Model file for the job. Use its own axes, mm. Face numbers are marked on the shaded views. A direction names the side the tool comes from. Round coordinates to 2 decimals unless told otherwise and drop trailing zeros. Loops run counter-clockwise (first coordinate to the right, second up) from the corner with the lowest first, then second, coordinate; pieces in that order, holes last. Notation, with made-up numbers: (-23, 79) - (33, 79) arc R16 ccw to (33, 98) - close; hole circle Ø4 at (23.5, 1.25). An arc over 180 degrees is marked (long way). Answer as a JSON object with one key per item and string values.
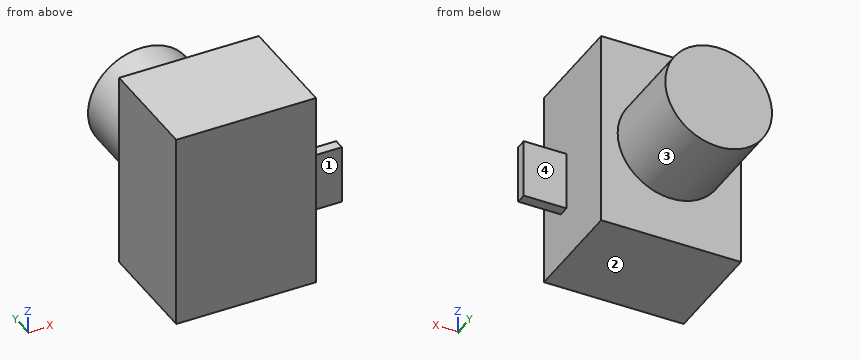
Autodesk Inventor part; units mm, degrees
ref_plane "YZ Plane" through (0, 0, 0) normal (1, 0, 0) x (0, 1, 0)
ref_plane "XZ Plane" through (0, 0, 0) normal (0, 1, 0) x (-1, 0, 0)
ref_plane "XY Plane" through (0, 0, 0) normal (0, 0, 1) x (1, 0, 0)
sketch "Sketch1" plane through (0, 0, 0) normal (0, 1, 0) x (-1, 0, 0)
  line L0 (-6.55, 9.3) -> (6.55, 9.3)
  line L1 (6.55, 9.3) -> (6.55, -9.3)
  line L2 (6.55, -9.3) -> (-6.55, -9.3)
  line L3 (-6.55, -9.3) -> (-6.55, 9.3)
  line L4 (0, 0) -> (1, 0)
  line L5 (0, 0) -> (0, -1)
  dimension "d0" = 18.6
  dimension "d1" = 13.1
  dimension "d2" = 1
  dimension "d3" = 1
extrude "Extrusion1" add sketch "Sketch1" along normal blind 10.2
sketch "Sketch2" plane through (0, 10.2, 0) normal (0, 1, 0) x (1, 0, 0)
  circle A0 centre (0, 0) radius 5
  dimension "d6" = 10
extrude "Extrusion2" add sketch "Sketch2" along normal blind 8.5
sketch "Sketch3" plane through (6.55, 0, 9.3) normal (1, 0, 0) x (0, 0, -1)
  point P0 (9.3, 0)
sketch "Sketch4" plane through (6.55, 0, 9.3) normal (1, 0, 0) x (0, 0, -1)
  circle A0 centre (7.5, 3.5) radius 2.5
  line L0 (0, 0) -> (0, 10.2)
  line L1 (18.6, 0) -> (0, 0)
  point P0 (9.3, 0)
  dimension "d9" = 5
  dimension "d10" = 7.5
  dimension "d11" = 3.5
extrude "Extrusion3" [suppressed]
sketch "Sketch5" plane through (11.55, 3.5, 1.8) normal (1, 0, 0) x (0, 0, -1)
  circle A0 centre (0, 0) radius 15
  point P0 (1.8, -3.5)
  dimension "d14" = 30
extrude "Extrusion4" [suppressed]
sketch "Náčrt6" plane through (6.55, 0, 9.3) normal (1, 0, 0) x (0, 0, -1)
  line L0 (18.6, 0) -> (0, 0)
  line L1 (18.6, 0) -> (18.6, 10.2)
  line L2 (0, 10.2) -> (18.6, 10.2)
  line L3 (0, 0) -> (0, 10.2)
  line L4 (13.6, 3) -> (8.1, 3)
  line L5 (8.1, 3) -> (8.1, 4)
  line L6 (8.1, 4) -> (13.6, 4)
  line L7 (13.6, 4) -> (13.6, 3)
  point P0 (9.3, 0)
  dimension "d17" = 10.2
  dimension "d18" = 18.6
  dimension "d19" = 3
  dimension "d20" = 1
  dimension "d21" = 5.5
  dimension "d22" = 5
extrude "Vysunutí5" add sketch "Náčrt6" along normal blind 4 contours L4 L5 L6 L7
properties part number "Camera"
1) Probe probe 1 along X at (y, z) = (10.25, 0); probe 2 along Y at (x, z) = (1.5, 7); probe 3 along Y at (x, z) = (9.5, -1.5). List the from-to ranges inside material, lowest first.
Values follow:
{"probe 1": "-5 to 5", "probe 2": "0 to 10.2", "probe 3": "3 to 4"}
2) Slice it at D-D on x = -3. List the corners of the cut face in (y, z).
Values follow:
{"outline": "(0, -9.3) - (10.2, -9.3) - (10.2, -4) - (18.7, -4) - (18.7, 4) - (10.2, 4) - (10.2, 9.3) - (0, 9.3) - close"}
3) Slice it at A-A on x = 0. List the corners of the cut face in (y, z).
Values follow:
{"outline": "(0, -9.3) - (10.2, -9.3) - (10.2, -5) - (18.7, -5) - (18.7, 5) - (10.2, 5) - (10.2, 9.3) - (0, 9.3) - close"}
4) Slice it at B-B on z = 0. List the corners of the cut face in (x, y).
Values follow:
{"outline": "(-6.55, 0) - (6.55, 0) - (6.55, 3) - (10.55, 3) - (10.55, 4) - (6.55, 4) - (6.55, 10.2) - (5, 10.2) - (5, 18.7) - (-5, 18.7) - (-5, 10.2) - (-6.55, 10.2) - close"}
5) Slice it at C-C on y = 13. List the corners of the cut face in (x, z), then the cut area to 3 significant figures.
Values follow:
{"outline": "circle Ø10 at (0, 0)", "area": "78.5 mm²"}
6) Drop flat-ended pins along their axis: P1, Ø0.8, axis at x = 9, y = 3.5, coming from the -Z side; P2, Ø10, axis at y = 9, z = -5.5, coming from the +X side; P3, Ø2, axis at x = 8.5, z = -2, coming from the -Y side. Give the stop position or say it passes through.
Values follow:
{"P1": "z = -4.3", "P2": "x = 6.55", "P3": "y = 3"}
7) Tool access for the marked faces 1, 2, 3 and 4: list every direction of +Z, -Z, +X, -X, +Y, -Y with a clear straight run to the whole face (end or side of a thin tool).
Values follow:
{"face 1": "+Z, -Z, +X, -Y", "face 2": "-Z, +X, -X, +Y, -Y", "face 3": "+Y", "face 4": "+Z, -Z, +X, +Y"}
